Autodesk Inventor part; units mm, degrees
ref_plane "YZ Plane" through (0, 0, 0) normal (1, 0, 0) x (0, 1, 0)
ref_plane "XZ Plane" through (0, 0, 0) normal (0, 1, 0) x (-1, 0, 0)
ref_plane "XY Plane" through (0, 0, 0) normal (0, 0, 1) x (1, 0, 0)
sketch "Sketch1" plane through (0, 0, 0) normal (1, 0, 0) x (0, 1, 0)
  line L0 (0, 0) -> (35, 0)
  line L1 (35, 0) -> (35, 27)
  line L2 (35, 27) -> (0, 27)
  line L3 (0, 27) -> (0, 0)
  line L4 (0, 27) -> (25, 27) construction
  line L5 (25, 27) -> (25, 0) construction
  line L6 (25, 0) -> (0, 0) construction
  line L7 (0, 0) -> (0, 27) construction
  circle A0 centre (12.5, 12.5) radius 6.35
  dimension "d0" = 35
  dimension "d1" = 27
  dimension "d2" = 25
  dimension "d3" = 12.7
extrude "Extrusion1" add sketch "Sketch1" along normal blind 10
sketch "Sketch2" plane through (10, 0, 0) normal (1, 0, 0) x (0, 0, -1)
  line L0 (0, 35) -> (-27, 35)
  line L1 (0, 0) -> (0, 35)
  line L2 (-27, 35) -> (0, 35)
  line L3 (0, 35) -> (0, 25)
  line L4 (0, 25) -> (-27, 25)
  line L5 (-27, 25) -> (-27, 35)
  dimension "d6" = 10
extrude "Extrusion2" add sketch "Sketch2" along normal blind 10
sketch "Sketch3" plane through (10, 0, 0) normal (1, 0, 0) x (0, 0, -1)
  point P0 (0, 0)
sketch "Sketch4" plane through (0, 0, 0) normal (0, 0, -1) x (-1, 0, 0)
  point P0 (0, 0)
sketch "Sketch5" plane through (10, 0, 0) normal (1, 0, 0) x (0, 0, -1)
  point P0 (0, 0)
sketch "Sketch6" plane through (10, 0, 0) normal (1, 0, 0) x (0, 0, -1)
  line L0 (-27, 25) -> (-27, 0)
  line L1 (-27, 0) -> (-22, 0)
  line L2 (-22, 0) -> (-22, 11)
  line L3 (-22, 11) -> (-27, 11)
  line L4 (-27, 11) -> (-27, 0)
  line L5 (-22, 14) -> (-27, 14)
  line L6 (-27, 14) -> (-27, 19)
  line L7 (-27, 19) -> (-22, 19)
  line L8 (-22, 19) -> (-22, 14)
  point P0 (0, 0)
  dimension "d9" = 5
  dimension "d10" = 11
  dimension "d11" = 5
extrude "Extrusion3" add sketch "Sketch6" along normal blind 150
sketch "Sketch7" plane through (10, 19, 27) normal (0, 1, 0) x (1, 0, 0)
  line L0 (-10, 0) -> (10, 0)
  line L1 (0, 5) -> (150, 5)
  line L2 (0, 0) -> (10, 0)
  line L3 (10, 0) -> (10, 5)
  line L4 (10, 5) -> (0, 5)
  line L5 (0, 5) -> (0, 0)
  point P0 (-10, 27)
  dimension "d14" = 10
extrude "Extrusion4" add sketch "Sketch7" along normal blind 7.5
sketch "Sketch8" plane through (160, 0, 0) normal (1, 0, 0) x (0, 0, -1)
  line L0 (-27, 14) -> (-22, 14)
  line L1 (-27, 14) -> (-22, 14)
  line L2 (-22, 25) -> (-22, 14)
  line L3 (-22, 14) -> (-22, 25)
  line L4 (-22, 25) -> (0, 25)
  line L5 (-22, 25) -> (0, 25)
  line L6 (0, 25) -> (0, 35)
  line L7 (0, 25) -> (0, 35)
  line L8 (0, 35) -> (-27, 35)
  line L9 (-27, 35) -> (-27, 14)
  line L10 (-22, 11) -> (-22, 0)
  line L11 (-27, 0) -> (-22, 0)
  line L12 (-22, 0) -> (-22, 11)
  line L13 (-22, 11) -> (-27, 11)
  line L14 (-27, 11) -> (-27, 0)
  point P0 (0, 0)
extrude "Extrusion5" add sketch "Sketch8" along normal blind 10
sketch "Sketch9" plane through (170, 0, 0) normal (1, 0, 0) x (0, 0, -1)
  line L0 (0, 35) -> (-27, 35)
  line L1 (-27, 35) -> (0, 35)
  line L2 (0, 35) -> (0, 0)
  line L3 (0, 0) -> (-27, 0)
  line L4 (-27, 0) -> (-27, 35)
  circle A0 centre (-12.5, 12.5) radius 6.35
  circle A1 centre (-12.5, 12.5) radius 6.35
extrude "Extrusion6" add sketch "Sketch9" along normal blind 10
fillet "Fillet1" radius 2 2 edges at (90, 11, 22) (90, 14, 22)
sketch "Sketch10" plane through (20, 0, 0) normal (1, 0, 0) x (0, 0, -1)
  line L0 (0, 35) -> (-27, 35)
  line L1 (-13.5, 35) -> (-20.5, 35)
  line L2 (-20.5, 35) -> (-6.5, 35)
  line L3 (-20.5, 35) -> (-6.5, 35)
  line L4 (-6.5, 35) -> (-6.5, 32)
  line L5 (-6.5, 32) -> (-20.5, 32)
  line L6 (-20.5, 32) -> (-20.5, 35)
  point P0 (0, 0)
  dimension "d22" = 7
  dimension "d23" = 14
  dimension "d24" = 3
extrude "Extrusion7" add sketch "Sketch10" along normal blind 140
sketch "Sketch11" plane through (0, 35, 27) normal (0, 1, 0) x (1, 0, 0)
  point P0 (0, 27)
sketch "Sketch12" plane through (160, 25, 0) normal (0, 0, -1) x (-1, 0, 0)
  line L0 (-4, 3.5) -> (-16, 3.5)
  line L1 (-16, 3.5) -> (-16, 6.5)
  line L2 (-16, 6.5) -> (-4, 6.5)
  line L3 (-4, 6.5) -> (-4, 3.5)
  line L4 (-4, 3.5) -> (-16, 6.5) construction
  line L5 (-16, 3.5) -> (-4, 6.5) construction
  line L6 (156, 6.5) -> (144, 6.5)
  line L7 (144, 6.5) -> (144, 3.5)
  line L8 (144, 3.5) -> (156, 3.5)
  line L9 (156, 3.5) -> (156, 6.5)
  line L10 (156, 6.5) -> (144, 3.5) construction
  line L11 (144, 6.5) -> (156, 3.5) construction
  point P0 (160, -25)
  point P1 (-10, 5)
  point P2 (150, 5)
  dimension "d27" = 12
  dimension "d28" = 3
  dimension "d29" = 12
  dimension "d30" = 3
extrude "Extrusion8" cut sketch "Sketch12" against normal blind 23.5
sketch "Sketch13" plane through (0, 0, 0) normal (-1, 0, 0) x (0, 0, 1)
  circle A0 centre (12.5, 12.5) radius 6.35 construction
  circle A1 centre (12.5, 12.5) radius 20.6375 construction
  point P0 (0, 0)
  dimension "d33" = 41.275
sketch "Sketch14" plane through (170, 0, 0) normal (-1, 0, 0) x (0, 0, 1)
  circle A0 centre (12.5, 12.5) radius 6.35
  circle A1 centre (12.5, 12.5) radius 6.35
  circle A2 centre (12.5, 12.5) radius 3.5
  point P0 (0, 0)
  dimension "d34" = 7
extrude "Extrusion9" add sketch "Sketch14" against normal blind 4.5
sketch "Sketch15" plane through (10, 0, 0) normal (1, 0, 0) x (0, 0, -1)
  circle A0 centre (-12.5, 12.5) radius 3.5
  circle A1 centre (-12.5, 12.5) radius 6.35
  circle A2 centre (-12.5, 12.5) radius 3.5
  point P0 (0, 0)
  dimension "d37" = 7
extrude "Extrusion10" add sketch "Sketch15" against normal blind 4.5
sketch "Sketch16" plane through (0, 0, 27) normal (0, 0, 1) x (1, 0, 0)
  point P0 (0, 0)
sketch "Sketch17" plane through (0, 0, 27) normal (0, 0, 1) x (1, 0, 0)
  point P0 (0, 0)
sketch "Sketch18" plane through (0, 0, 27) normal (0, 0, 1) x (1, 0, 0)
  line L0 (0, 35) -> (0, 0)
  line L1 (180, 35) -> (180, 0)
  line L2 (0, 0) -> (180, 0)
  line L3 (180, 0) -> (180, 3)
  line L4 (180, 3) -> (0, 3)
  line L5 (0, 3) -> (0, 0)
  point P0 (0, 3)
  dimension "d40" = 3
extrude "Extrusion11" add sketch "Sketch18" against normal blind 67
sketch "Sketch19" plane through (0, 3, 27) normal (0, 1, 0) x (-1, 0, 0)
  line L0 (180, 0) -> (180, -42) construction
  point P0 (0, 0)
sketch "Sketch20" plane through (0, 3, -40) normal (0, 1, 0) x (1, 0, 0)
  circle A0 centre (90, -20) radius 19
  circle A1 centre (90, -20) radius 20
  circle A2 centre (50, -20) radius 20
  circle A3 centre (50, -20) radius 19
  circle A4 centre (130, -20) radius 20
  circle A5 centre (130, -20) radius 19
  point P0 (0, -40)
  point P1 (110, -20)
  point P2 (70, -20)
  dimension "d43" = 38
  dimension "d44" = 38
  dimension "d45" = 38
extrude "Extrusion12" add sketch "Sketch20" along normal blind 30
sketch "Sketch21" plane through (10, 3, 22) normal (0, 1, 0) x (1, 0, 0)
  line L0 (-10, 22) -> (-10, 62)
  line L1 (-10, 62) -> (10, 62)
  line L2 (10, 62) -> (10, 52)
  line L3 (10, 52) -> (-10, 52)
  line L4 (-10, 52) -> (-10, 62)
  line L5 (170, 62) -> (-10, 62)
  line L6 (170, 62) -> (150, 62)
  line L7 (150, 62) -> (150, 52)
  line L8 (150, 52) -> (170, 52)
  line L9 (170, 52) -> (170, 62)
  dimension "d48" = 10
  dimension "d49" = 10
extrude "Extrusion13" add sketch "Sketch21" along normal blind 32
sketch "Sketch22" plane through (4, 28.5, 0) normal (0, 1, 0) x (1, 0, 0)
  point P0 (-4, 0)
sketch "Sketch23" plane through (0, 0, -40) normal (0, 0, -1) x (-1, 0, 0)
  line L0 (-4, 28.5) -> (-16, 28.5)
  line L1 (-4, 31.5) -> (-4, 28.5)
  line L2 (-16, 28.5) -> (-4, 28.5)
  line L3 (-4, 28.5) -> (-4, 31.5)
  line L4 (-4, 31.5) -> (-16, 31.5)
  line L5 (-16, 31.5) -> (-16, 28.5)
  line L6 (-164, 28.5) -> (-176, 28.5)
  line L7 (-164, 31.5) -> (-164, 28.5)
  line L8 (-176, 28.5) -> (-164, 28.5)
  line L9 (-164, 28.5) -> (-164, 31.5)
  line L10 (-164, 31.5) -> (-176, 31.5)
  line L11 (-176, 31.5) -> (-176, 28.5)
  point P0 (0, 0)
extrude "Extrusion14" cut sketch "Sketch23" against normal blind 10
sketch "Sketch24" plane through (130, 33, -20) normal (0, 1, 0) x (1, 0, 0)
  line L0 (27.2959, -23.1323) -> (-103.8128, -23.1323)
  line L1 (-103.8128, -23.1323) -> (-103.8128, 25.7271)
  line L2 (-103.8128, 25.7271) -> (27.2959, 25.7271)
  line L3 (27.2959, 25.7271) -> (27.2959, -23.1323)
  point P0 (-130, -20)
extrude "Extrusion15" cut sketch "Sketch24" against normal blind 30
sketch "Sketch25" plane through (10, 3, 22) normal (0, 1, 0) x (1, 0, 0)
  circle A0 centre (80, 38.75) radius 19
  circle A1 centre (80, 38.75) radius 20.75
  circle A2 centre (121.5, 38.75) radius 20.75
  circle A3 centre (121.5, 38.75) radius 19
  circle A4 centre (38.5, 38.75) radius 20.75
  circle A5 centre (38.5, 38.75) radius 19
  point P0 (-10, 22)
  point P1 (59.25, 38.75)
  point P2 (100.75, 38.75)
  dimension "d56" = 38
  dimension "d57" = 41.5
  dimension "d58" = 38
  dimension "d59" = 38
extrude "Extrusion16" add sketch "Sketch25" along normal blind 45
sketch "Sketch26" plane through (0, 35, 27) normal (0, 1, 0) x (1, 0, 0)
  line L0 (20, 6.5) -> (160, 6.5)
  line L1 (20, 20.5) -> (160, 20.5)
  line L2 (20, 6.5) -> (160, 6.5)
  line L3 (160, 6.5) -> (160, 20.5)
  line L4 (160, 20.5) -> (20, 20.5)
  line L5 (20, 20.5) -> (20, 6.5)
  point P0 (0, 27)
extrude "Extrusion17" cut sketch "Sketch26" against normal blind 5
properties part number "_3DPrint"
Model file for the job. Use its own axes, mm. A direction names the side the tool comes from. Give positions to 0.01 mm unless a question says otherwise; leave off trailing zeros. Order: outer loops, then holes, each group sorted by start corner. A loop starts at its lowest first (then second) coordinate and runs counter-clockwise, first axis right, second up. Notation, with made-up numbers: M -6,70.5 L 2,70.5 A8 ccw 2,75.5 Z; hole C -21,65 d4. An arc over 180 degrees is marked long. Put each result on its own line as item: value. Start each with the question number.
(1) Pin check, flat tips, straight feed: pin 1 Ø5 at (x, z) = (34, -17) entering from +Y; pin 2 Ø1.5 at (y, z) = (15, 10.5) entering from -X; pin 3 Ø3.5 at (x, z) = (109, 25.5) entering from +Y. Stop position of each tip, or through.
(2) Tool access for faces 4 (the face through (2.712, 15.43, 18.134)), 5 (the face through (49, 3, -16)), 6 (the face through (10, 28.5, 12)), 7 (the face through (20, 29, 14)): list every direction of +Z, -Z, +X, -X, +Y, -Y with a clear straight run to the whole face (end or side of a thin tool).
(3) Band-saw the part on D-D on x = 48.5. Give the cut face in (y, z), then the cut area to 3 significant figures.
(4) Pull direction X, two halves, no side cores. Call faces 1 (the face through (172, 23, 0)), 2 (the face through (90, 25, 4)), 3 (the face through (16, 30, -35)): released by +X, released by -X, zero draft, split by the parting line, or undercut.
(5) Band-saw the part on B-B on x = 166.5. Give the cut face in (y, z).
(6) Drill centre lines: L1, parallel to Z at x = 3.9, y = 12.5; L2, parallel to Z at x = 15, y = 33; L3, parallel to X at y = 36, z = -19. Where is each one in solid material? Low to high. Write a range as [from, to].
Results below:
1. pin 1: stops at y = 3
1. pin 2: stops at x = 5.5
1. pin 3: stops at y = 19
2. face 4: -X
2. face 5: +Y
2. face 6: -Z
2. face 7: +Z, -Z, +Y
3. outline: M 0,-40 L 3,-40 L 3,-37.5 L 48,-37.5 L 48,-35.75 L 3,-35.75 L 3,2.25 L 48,2.25 L 48,4 L 3,4 L 3,22 L 9,22 A2 ccw 11,24 L 11,27 L 0,27 Z; M 14,24 A2 ccw 16,22 L 19,22 L 19,27 L 14,27 Z
3. area: 422 mm2
4. face 1: zero draft
4. face 2: undercut
4. face 3: undercut
5. outline: M 0,-40 L 28.5,-40 L 28.5,-30 L 3,-30 L 3,22 L 9,22 A2 ccw 11,24 L 11,27 L 0,27 Z; M 14,24 A2 ccw 16,22 L 25,22 L 25,0 L 28.5,0 L 28.5,23.5 L 31.5,23.5 L 31.5,0 L 35,0 L 35,27 L 14,27 Z; M 31.5,-40 L 35,-40 L 35,-30 L 31.5,-30 Z
6. L1: z = [-40, -30], [0, 6.15], [18.85, 27]
6. L2: z = [-40, -30], [0, 27]
6. L3: x = [27.87, 29.63], [67.37, 69.13], [69.37, 71.13], [108.87, 110.63], [110.87, 112.63], [150.37, 152.13]
